Work out the finished part from the listing and answer in its coordinate system (mm). A direction names the side the tool comes from. Give positions to 0.01 mm unless a question says otherwise; leave off trailing zeros. Loops run counter-clockwise (first coordinate to the right, second up) from the corner with the lowest first, then second, coordinate; pieces in that order, holes last. Notation, with made-up numbers: M -12.75,-14.5 L 2.25,-14.5 A35 ccw 2.25,22.5 Z; hole C -3,25 d10. An arc over 180 degrees is marked long. Use a Markdown table: item, result.
```python
from build123d import *

# Parameters (mm, degrees)
BOSS_EXTRUDE1_DEPTH = 2.58
CUT_EXTRUDE1_DEPTH  = 10.5
CUT_EXTRUDE2_DEPTH  = 5.25
BOSS_EXTRUDE2_DEPTH = 0.5
CHAMFER1_SIZE       = 0.6
CHAMFER2_SIZE       = 0.4


with BuildPart() as part:
    # Sketch1 → Boss-Extrude1 (new body)
    with BuildSketch(Plane.XY):
        with BuildLine():
            Line((-2.75, -4), (-2.75, 4.05))
            ThreePointArc((-2.75, 4.05), (-2.544974747, 4.544974747), (-2.05, 4.75))
            Line((-2.05, 4.75), (2.05, 4.75))
            ThreePointArc((2.05, 4.75), (2.544974747, 4.544974747), (2.75, 4.05))
            Line((2.75, 4.05), (2.75, -4))
            Line((2.75, -4), (2.25, -4))
            Line((2.25, -4), (2.25, 4.05))
            ThreePointArc((2.25, 4.05), (2.191421356, 4.191421356), (2.05, 4.25))
            Line((2.05, 4.25), (-2.05, 4.25))
            ThreePointArc((-2.05, 4.25), (-2.191421356, 4.191421356), (-2.25, 4.05))
            Line((-2.25, 4.05), (-2.25, -4))
            Line((-2.25, -4), (-2.75, -4))
        make_face()
    extrude(amount=BOSS_EXTRUDE1_DEPTH)

    # Sketch2 → Cut-Extrude1 (cut)
    with BuildSketch(Plane(origin=(0, 4.75, 0), x_dir=(1, 0, 0), z_dir=(0, 1, 0))):
        Polygon((-2, -0.58), (-4.099439411, -0.58), (-4.099439411, 0.833357165), (-2, 0.833357165), (-1.6, 0), align=None)
        Polygon((2, -0.58), (3.357409655, -0.58), (3.357409655, 0.833357165), (2, 0.833357165), (1.6, 0), align=None)
        with BuildLine():
            Line((-2.75, -2.58), (-2.38062097, -2.58))
            ThreePointArc((-2.38062097, -2.58), (-2.104839164, -2.497066416), (-1.920543652, -2.275777582))
            Line((-1.920543652, -2.275777582), (-1.314728174, -0.852111209))
            ThreePointArc((-1.314728174, -0.852111209), (-1.222580418, -0.741466792), (-1.084689515, -0.7))
            Line((-1.084689515, -0.7), (1.084290526, -0.7))
            ThreePointArc((1.084290526, -0.7), (1.222412736, -0.741619926), (1.314545856, -0.852621958))
            Line((1.314545856, -0.852621958), (1.915985292, -2.274756083))
            ThreePointArc((1.915985292, -2.274756083), (2.100251533, -2.496760148), (2.376495952, -2.58))
            Line((2.376495952, -2.58), (2.75, -2.58))
            Line((2.75, -2.58), (2.75, -3.056093585))
            Line((2.75, -3.056093585), (-2.75, -3.056093585))
            Line((-2.75, -3.056093585), (-2.75, -2.58))
        make_face()
    extrude(amount=-CUT_EXTRUDE1_DEPTH, mode=Mode.SUBTRACT)

    # Sketch3 → Cut-Extrude2 (cut, symmetric)
    with BuildSketch(Plane(origin=(0, 0, 0), x_dir=(0, 0, -1), z_dir=(1, 0, 0))):
        Polygon((-0.58, 0.25), (-1.08, -0.35), (-1.08, -4.396314828), (-0.130305992, -4.396314828), (-0.130305992, 0.25), align=None)
        Polygon((-2.58, 0.25), (-2.08, -0.35), (-2.08, -4.896314828), (-3.070294312, -4.896314828), (-3.070294312, 0.25), align=None)
        with BuildLine():
            Line((-1.08, 3.024565065), (-1.08, 1.024565065))
            ThreePointArc((-1.08, 1.024565065), (-1.58, 0.524565065), (-2.08, 1.024565065))
            Line((-2.08, 1.024565065), (-2.08, 3.024565065))
            ThreePointArc((-2.08, 3.024565065), (-1.58, 3.524565065), (-1.08, 3.024565065))
        make_face()
    extrude(amount=CUT_EXTRUDE2_DEPTH, both=True, mode=Mode.SUBTRACT)

    # Sketch4 → Boss-Extrude2 (add, symmetric)
    with BuildSketch(Plane(origin=(0, 0, 0), x_dir=(0, 0, -1), z_dir=(1, 0, 0))):
        with BuildLine():
            Line((-0.7, 4.25), (-1.045169213, 3.954140675))
            ThreePointArc((-1.045169213, 3.954140675), (-1.420160684, 3.782160221), (-1.829373497, 3.834512432))
            Line((-1.829373497, 3.834512432), (-2.4, 4.079724782))
            Line((-2.4, 4.079724782), (-2.202592831, 4.539105245))
            Line((-2.202592831, 4.539105245), (-1.631966328, 4.293892895))
            ThreePointArc((-1.631966328, 4.293892895), (-1.495562057, 4.276442158), (-1.3705649, 4.333768976))
            Line((-1.3705649, 4.333768976), (-0.997308957, 4.653702641))
            ThreePointArc((-0.997308957, 4.653702641), (-0.875770907, 4.725154006), (-0.736992408, 4.75))
            Line((-0.736992408, 4.75), (-0.7, 4.75))
            Line((-0.7, 4.75), (-0.7, 4.25))
        make_face()
    extrude(amount=BOSS_EXTRUDE2_DEPTH, both=True)

    # Chamfer1
    chamfer1_edges = [part.edges().sort_by_distance(p)[0] for p in [
        (2.5, -4, 1.08),
        (-2.5, -4, 1.08),
    ]]
    chamfer(chamfer1_edges, length=CHAMFER1_SIZE)

    # Chamfer2
    chamfer2_edges = [part.edges().sort_by_distance(p)[0] for p in [
        (-2.5, -4, 2.08),
        (2.5, -4, 2.08),
    ]]
    chamfer(chamfer2_edges, length=CHAMFER2_SIZE - 0.0001)  # a hair under: the kernel refuses the full size


solid = part.part
```
(1) A cutting plane is placed at C-C (z = 0.4). Write down the section's boundary in (x, y), and give its area (3 significant figures).
Entries:
| item | result |
|---|---|
| outline | M -1.88,4.25 L 1.88,4.25 L 1.88,4.75 L -1.88,4.75 Z |
| area | 1.88 mm² |
(2) Consider probe 1 along X at (y, z) = (-0.5, 1.2); probe 2 along Z at (x, y) = (2.45, 2.5); probe 3 along Y at (x, z) = (1.6, 0.35). Determine where each line is inside the solid, lowest interval first. Write a range as [from, to].
Entries:
| item | result |
|---|---|
| probe 1 | x = [-2.75, -2.25], [2.25, 2.75] |
| probe 2 | z = [0.58, 1.08], [2.08, 2.58] |
| probe 3 | y = [4.25, 4.75] |
(3) Which of the six approach directions +Z, -Z, +X, -X, +Y, -Y give full straight-line access (tool end or side, diameter ignored) to faces 1 (the flat face through (-2.25, 0, 2)), 2 (the flat face through (0, 4.25, 0.4)), 3 (the flat face through (0.5, 4.16, 1.35))?
Entries:
| item | result |
|---|---|
| face 1 | +Z, -Z, -Y |
| face 2 | -Z, -Y |
| face 3 | +Z, +Y, -Y |
(4) A cutting plane is placed at B-B (y = 2). Write down the section's boundary in (x, z), and give its area (3 significant figures).
Entries:
| item | result |
|---|---|
| outline | M -2.75,0.58 L -2.25,0.58 L -2.25,1.08 L -2.75,1.08 Z; M -2.75,2.08 L -2.25,2.08 L -2.25,2.56 A0.5 ccw -2.38,2.58 L -2.75,2.58 Z; M 2.25,0.58 L 2.75,0.58 L 2.75,1.08 L 2.25,1.08 Z; M 2.25,2.08 L 2.75,2.08 L 2.75,2.58 L 2.38,2.58 A0.5 ccw 2.25,2.56 Z |
| area | 0.999 mm² |
(5) Given P1, Ø0.6, axis at x = 2.5, y = 1.5, coming from the -Z side; P2, Ø1.5, axis at x = 2, y = -2.5, coming from the -Z side; P3, Ø1.5, axis at x = -0.5, z = 2.5, coming from the +Y side, each flat-ended and moving along its own axis, determine where each tip first touches the part or whether it passes through.
Entries:
| item | result |
|---|---|
| P1 | stops at z = 0.58 |
| P2 | stops at z = 1.08 |
| P3 | stops at y = 4.54 |
(6) A cutting plane is placed at A-A (y = -1.25). Write down the section's boundary in (x, z).
Entries:
| item | result |
|---|---|
| outline | M -2.75,1.08 L -2.25,1.08 L -2.25,2.08 L -2.75,2.08 Z; M 2.25,1.08 L 2.75,1.08 L 2.75,2.08 L 2.25,2.08 Z |
(7) The mould has two halves that part along X. Classify faces 4 (the flat face through (-0.5, 4.16, 1.35)), 5 (the flat face through (2.25, 0, 2)), 6 (the flat face through (2.75, 0, 2)), 7 (the flat face through (-2.75, 0, 2)): released by +X, released by -X, zero draft, split by the parting line, or undercut.
Entries:
| item | result |
|---|---|
| face 4 | undercut |
| face 5 | undercut |
| face 6 | released by +X |
| face 7 | released by -X |
